Can you work these out from the model? Positions are in its coordinate system, mm. Face numbers are marked on the shaded views. A direction names the side the tool comes from. Give positions to 0.01 mm unless a question says otherwise; leave off trailing zeros. Loops run counter-clockwise (first coordinate to the right, second up) from the corner with the lowest first, then second, coordinate; pieces in that order, holes last.
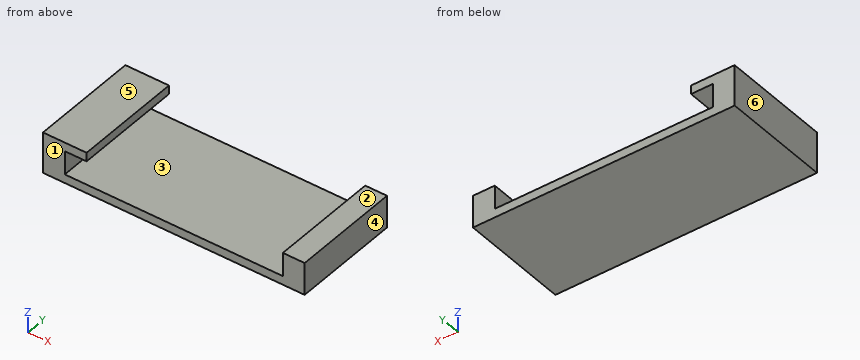
from build123d import *

# Parameters (mm, degrees)
F0_W     = 6.35
F0_H     = 31.75
F0_W_2   = 63.5
F1_DEPTH = 2.54
F2_DEPTH = 9.398
F3_W     = 6.35
F3_H     = 31.75
F4_DEPTH = 2.54


with BuildPart() as f1:
    # F0 (on Top) → F1 (new body)
    with BuildSketch(Plane.XY):
        with Locations((-34.925, 15.875)):
            Rectangle(F0_W, F0_H)
        with Locations((0, 15.875)):
            Rectangle(F0_W_2, F0_H)
        with Locations((34.925, 15.875)):
            Rectangle(F0_W, F0_H)
    extrude(amount=F1_DEPTH)

    # F0 (on Top) → F2 (join)
    with BuildSketch(Plane.XY):
        with Locations((-34.925, 15.875)):
            Rectangle(F0_W, F0_H)
        with Locations((34.925, 15.875)):
            Rectangle(F0_W, F0_H)
    extrude(amount=F2_DEPTH)

    # F3 (on face) → F4 (join)
    with BuildSketch(Plane.XY.offset(9.398)):
        with Locations((-28.575, 15.875)):
            Rectangle(F3_W, F3_H)
        with Locations((-34.925, 15.875)):
            Rectangle(F3_W, F3_H)
    extrude(amount=F4_DEPTH)


solid = f1.part
(1) Suppose I cut it at D-D on z = 10.5. List the corners of the cut face in (x, y) for me, plus the area to 3 significant figures.
Returned:
outline: (-38.1, 0) - (-25.4, 0) - (-25.4, 31.75) - (-38.1, 31.75) - close
area: 403 mm2
(2) Which directions (+Z, -Z, +X, -X, +Y, -Y) give clear straight access to the entire face, cutting with the end or side of a thin tool? Please do the marked faces 1 and 2.
Returned:
face 1: +Z, -Z, +X, -X, -Y
face 2: +Z, +X, +Y, -Y
(3) Will these pins go through, and if not, where does the flat tip stop? P1, Ø3, axis at y = 12, z = 11, coming from the +X side; P2, Ø3, axis at x = 35, y = 11, coming from the +Z side; P3, Ø2, axis at x = -24, z = 7.5, coming from the -Y side.
Returned:
P1: stops at x = -25.4
P2: stops at z = 9.4
P3: passes through
(4) Suppose I cut it at C-C on y = 8. List the corners of the cut face in (x, z) for me, plus the area to 3 significant figures.
Returned:
outline: (-38.1, 0) - (38.1, 0) - (38.1, 9.4) - (31.75, 9.4) - (31.75, 2.54) - (-31.75, 2.54) - (-31.75, 9.4) - (-25.4, 9.4) - (-25.4, 11.94) - (-38.1, 11.94) - close
area: 313 mm2
(5) Please list where these lines run through material, in increasing order: probe 1 along X at (y, z) = (24.5, 6.75); probe 2 along Z at (x, y) = (-26, 10.5).
Returned:
probe 1: x = -38.1 to -31.75, 31.75 to 38.1
probe 2: z = 0 to 2.54, 9.4 to 11.94
(6) Thinking about a two-plate mould opening in X: for the marked faces 3, 4, 5 and 6, which applies, pulls with the +X half, pulls with the -X half, needs draft (parallel to the pull), parting line crosses it, or undercut?
Returned:
face 3: undercut
face 4: pulls with the +X half
face 5: needs draft
face 6: pulls with the -X half
(7) Suppose I cut it at B-B on x = -28. List the corners of the cut face in (y, z) for me, plus the area to 3 significant figures.
Returned:
outline: (0, 0) - (31.75, 0) - (31.75, 2.54) - (0, 2.54) - close; (0, 9.4) - (31.75, 9.4) - (31.75, 11.94) - (0, 11.94) - close
area: 161 mm2
(8) Suppose I cut it at A-A on z = 7. List the corners of the cut face in (x, y) for me.
Returned:
outline: (-38.1, 0) - (-31.75, 0) - (-31.75, 31.75) - (-38.1, 31.75) - close; (31.75, 0) - (38.1, 0) - (38.1, 31.75) - (31.75, 31.75) - close
